Read the model definition and answer for the solid it produces. Units are mm, in the model's axes. A direction names the side the tool comes from. Round coordinates to 2 decimals unless told otherwise and drop trailing zeros. Order: outer loops, then holes, each group sorted by start corner. A loop starts at its lowest first (then second) coordinate and runs counter-clockwise, first axis right, second up. Notation, with made-up numbers: (36.25, -6.5) - (50.25, -6.5) arc R14 cw to (50.25, -0.5) - close; hole circle Ø1 at (-25, 6). An arc over 180 degrees is marked (long way). One line per question, with ' | ' between items. Start each with the question number.
1) The mould has two halves that part along X. Classify faces 4 (the cylindrical face through (15.55, 4.89, 6.5)), 5 (the flat face through (10.16, 6, 0)), 6 (the conical face through (10.001, -11.676, 12.878)), 7 (the flat face through (19.05, -3, -12)): pulls with the +X half, pulls with the -X half, needs draft (parallel to the pull), parting line crosses it, or undercut.
2) The part is cut by section C-C, the plane x = -30.5. Give the vertices of the cut face in (y, z), plus the area to 3 significant figures.
3) For faces 1 (the flat face through (-25.72, 7, 0)), 2 (the conical face through (12.541, -11.676, 12.878)), 3 (the cylindrical face through (-12.88, 4.78, -2.75)), determine the directions among +Z, -Z, +X, -X, +Y, -Y from which every point of the face is accessible in a straight line to the end or side of a thin tool.
4) Straight lines are drawn through the part: line 1 (Y direction, x = 3, z = 0); line 2 (Z direction, x = 3, y = -4.25); line 3 (Z direction, x = -43, y = 2.5). For each, find the intervals that lie inside material, in ascending order. Write a range as from..to.
5) Flat-ended cylindrical pins translate along their axes: pin 1 (8 mm diameter, centred on x = 7, z = 11, fed in from -Y); pin 2 (4 mm diameter, centred on x = 6, y = -4, fed in from -Z); pin 3 (8.5 mm diameter, centred on y = -10.5, z = 4.5, fed in from -X); pin 4 (2 mm diameter, centred on x = -0.5, z = 3.5, fed in from -Y). Find the tip coordinate at first contact, or state that the pin passes through.
from build123d import *

# Parameters (mm, degrees)
CHAMFER1_SIZE  = 0.79375
CHAMFER1_SIZE2 = 3.175


with BuildPart() as part:
    # Esquisse1 → Revolution1 (revolve)
    with BuildSketch(Plane.XY, mode=Mode.PRIVATE) as revolution1_sk:
        Polygon((-45.72, 5.08), (19.05, 5.08), (19.05, 6.477), (15.24, 6.477), (15.24, 5.842), (12.7, 6.477), (12.7, 5.842), (10.16, 6.477), (10.16, 5.842), (7.62, 6.477), (7.62, 5.842), (5.08, 6.477), (-25.72, 6.477), (-25.72, 7.18), (-45.72, 7.18), align=None)
    revolve(revolution1_sk.sketch.rotate(Axis((0, -7.62, 0), (1, 0, 0)), 90), axis=Axis((0, -7.62, 0), (1, 0, 0)))

    # Chamfer1
    chamfer1_edges = [part.edges().sort_by_distance(p)[0] for p in [
        (19.05, -7.62, -14.097),
    ]]
    chamfer1_side = [part.faces().sort_by_distance(p)[0] for p in [
        (19.05, -7.62, -13.098723372),
    ]]
    chamfer(chamfer1_edges, length=CHAMFER1_SIZE, length2=CHAMFER1_SIZE2, reference=chamfer1_side[0])


solid = part.part
Values:
1) face 4: needs draft | face 5: undercut | face 6: undercut | face 7: pulls with the +X half
2) outline: circle Ø29.6 at (-7.62, 0); hole circle Ø25.4 at (-7.62, 0) | area: 181 mm^2
3) face 1: +X | face 2: none | face 3: +X, -X
4) line 1: y = -21.72..-20.32, 5.08..6.48 | line 2: z = -13.69..-12.24, 12.24..13.69 | line 3: z = -10.8..-7.67, 7.67..10.8
5) pin 1: stops at y = -19.83 | pin 2: stops at z = -13.98 | pin 3: passes through | pin 4: stops at y = -21.49
